Could you check a few things on this model? Use its own coordinates, in mm. Face numbers are marked on the shaded views. A direction names the side the tool comes from. Give positions to 0.01 mm unless a question says otherwise; leave off trailing zeros. Write each loop counter-clockwise with the first axis right and the second up, starting at its lowest first coordinate (ties: lowest second). Pieces come first, ordered by that corner, then holes. Notation, with made-up numbers: M 16.25,-10 L 32.25,-10 A37 cw 32.25,26 Z; hole C 0,82 d5. An arc over 180 degrees is marked long. Answer as CSV lines item,"result". Start each with the question number.
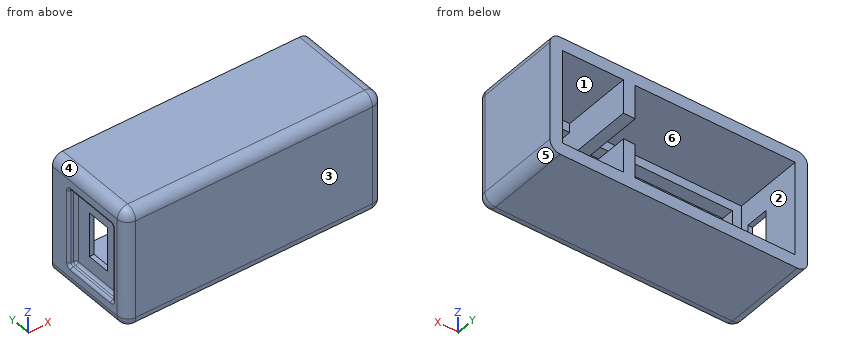
Autodesk Inventor part; units mm, degrees
ref_plane "YZ Plane" through (0, 0, 0) normal (1, 0, 0) x (0, 1, 0)
ref_plane "XZ Plane" through (0, 0, 0) normal (0, 1, 0) x (-1, 0, 0)
ref_plane "XY Plane" through (0, 0, 0) normal (0, 0, 1) x (1, 0, 0)
sketch "Sketch1" plane through (0, 0, 0) normal (0, 1, 0) x (-1, 0, 0)
  line L0 (0, 0) -> (-44.5, 0)
  line L1 (-44.5, 0) -> (-44.5, -18)
  line L2 (-44.5, -18) -> (0, -18)
  line L3 (0, -18) -> (0, 0)
  line L4 (2.4, -20.4) -> (-46.9, -20.4)
  line L5 (-46.9, -20.4) -> (-46.9, 2.4)
  line L6 (-46.9, 2.4) -> (2.4, 2.4)
  line L7 (2.4, 2.4) -> (2.4, -20.4)
  dimension "d0" = 18
  dimension "d1" = 44.5
  dimension "d2" = 2.4
extrude "Extrusion1" add sketch "Sketch1" against normal blind 2.4 contours L3 L2 L1 L0 | L4 L5 L6 L7
extrude "Extrusion2" add sketch "Sketch1" along normal blind 15.8
sketch "Sketch2" plane through (0, 0, 0) normal (0, 1, 0) x (1, 0, 0)
  line L0 (0, 0) -> (44.5, 0)
  line L1 (44.5, 0) -> (44.5, 18)
  line L2 (44.5, 18) -> (0, 18)
  line L3 (0, 18) -> (0, 0)
  line L4 (1.75, 16.25) -> (42.75, 16.25)
  line L5 (42.75, 16.25) -> (42.75, 1.75)
  line L6 (42.75, 1.75) -> (1.75, 1.75)
  line L7 (1.75, 1.75) -> (1.75, 16.25)
  line L8 (32.85, 17.25) -> (42.75, 17.25)
  line L9 (42.75, 17.25) -> (42.75, 0.75)
  line L10 (42.75, 0.75) -> (32.85, 0.75)
  line L11 (32.85, 0.75) -> (32.85, 17.25)
  line L12 (42.75, 13.5) -> (44.5, 13.5)
  line L13 (44.5, 13.5) -> (44.5, 4.5)
  line L14 (44.5, 4.5) -> (42.75, 4.5)
  line L15 (42.75, 4.5) -> (42.75, 13.5)
  line L16 (44.5, 18) -> (44.5, 0)
  point P0 (42.75, 9)
  point P1 (44.5, 9)
  point P2 (43.625, 4.5)
  point P3 (42.75, 4.5)
  point P4 (42.75, 13.5)
  dimension "d7" = 1.75
  dimension "d8" = 9.9
  dimension "d9" = 16.5
  dimension "d10" = 9
extrude "Extrusion3" add sketch "Sketch2" along normal blind 2.4 contours L3 L2 L1 L12 L5 L9 L8 L11 L4 L7 L6 L10 L14 L0 | L9 L10 L11 L6 | L4 L11 L8 L9
sketch "Sketch3" plane through (0, 2.4, 0) normal (0, 1, 0) x (1, 0, 0)
  line L0 (32.85, 0.75) -> (32.85, 17.25)
  line L1 (44.5, 4.5) -> (44.5, 0)
  line L2 (44.5, 4.5) -> (42.75, 4.5)
  line L3 (42.75, 4.5) -> (42.75, 1.75)
  line L4 (42.75, 1.75) -> (1.75, 1.75)
  line L5 (1.75, 1.75) -> (1.75, 16.25)
  line L6 (1.75, 16.25) -> (42.75, 16.25)
  line L7 (42.75, 16.25) -> (42.75, 13.5)
  line L8 (42.75, 13.5) -> (44.5, 13.5)
  line L9 (44.5, 18) -> (44.5, 13.5)
  line L10 (0, 18) -> (44.5, 18)
  line L11 (0, 0) -> (0, 18)
  line L12 (44.5, 0) -> (0, 0)
  line L13 (32.85, 18) -> (30.6, 18)
  line L14 (30.6, 18) -> (30.6, 11.5)
  line L15 (30.6, 11.5) -> (32.85, 11.5)
  line L16 (32.85, 11.5) -> (32.85, 18)
  line L17 (32.85, 0) -> (30.6, 0)
  line L18 (30.6, 0) -> (30.6, 6.5)
  line L19 (30.6, 6.5) -> (32.85, 6.5)
  line L20 (32.85, 6.5) -> (32.85, 0)
  line L21 (44.5, 0) -> (0, 0)
  line L22 (0, 18) -> (44.5, 18)
  point P0 (30.6, 1.75)
  point P1 (32.85, 1.75)
  point P2 (32.85, 16.25)
  point P3 (30.6, 16.25)
  point P4 (32.85, 0)
  dimension "d13" = 5
  dimension "d14" = 30.6
extrude "Extrusion4" add sketch "Sketch3" against normal up to surface (2.4 mm away) contours L0 L4 L18 L19 | L15 L14 L6 L0
extrude "Extrusion5" add sketch "Sketch3" along normal up to surface (13.4 mm away) contours L0 L4 L18 L19 | L15 L14 L6 L0 | L0 L20 L12 L18 L4 | L6 L14 L10 L16 L0
sketch "Sketch4" plane through (0, 2.4, 0) normal (0, 1, 0) x (1, 0, 0)
  line L0 (32.85, 18) -> (32.85, 16.25)
  line L1 (32.85, 16.25) -> (42.75, 16.25)
  line L2 (42.75, 16.25) -> (42.75, 13.5)
  line L3 (42.75, 13.5) -> (44.5, 13.5)
  line L4 (44.5, 18) -> (44.5, 13.5)
  line L5 (32.85, 18) -> (44.5, 18)
  line L6 (32.85, 1.75) -> (32.85, 0)
  line L7 (44.5, 0) -> (32.85, 0)
  line L8 (44.5, 4.5) -> (44.5, 0)
  line L9 (44.5, 4.5) -> (42.75, 4.5)
  line L10 (42.75, 4.5) -> (42.75, 1.75)
  line L11 (42.75, 1.75) -> (32.85, 1.75)
  line L12 (42.75, 16.25) -> (42.75, 18)
  line L13 (42.75, 1.75) -> (42.75, 0)
  point P0 (0, 0)
extrude "Extrusion6" add sketch "Sketch4" along normal blind 4.8 contours L5 L4 L3 L2 L12 | L10 L9 L8 L7 L13
sketch "Sketch5" plane through (-2.4, -2.4, -20.4) normal (-1, 0, 0) x (0, 0, 1)
  line L0 (20.4, 4.8) -> (2.4, 4.8)
  line L1 (7.15, 10.9) -> (15.65, 10.9)
  line L2 (15.65, 10.9) -> (15.65, 6.4)
  line L3 (15.65, 6.4) -> (7.15, 6.4)
  line L4 (7.15, 6.4) -> (7.15, 10.9)
  line L5 (11.4, 4.8) -> (11.4, 2.8169) construction
  point P0 (20.4, 2.4)
  point P1 (11.4, 6.4)
  dimension "d21" = 8.5
  dimension "d22" = 4.5
  dimension "d23" = 1.6
extrude "Extrusion7" cut sketch "Sketch5" against normal up to surface (2.4 mm away)
sketch "Sketch6" plane through (-2.4, -2.4, -20.4) normal (-1, 0, 0) x (0, 0, 1)
  line L0 (7.15, 10.9) -> (15.65, 10.9)
  line L1 (7.15, 6.4) -> (7.15, 10.9)
  line L2 (15.65, 6.4) -> (7.15, 6.4)
  line L3 (15.65, 10.9) -> (15.65, 6.4)
  line L4 (18.9, 14.15) -> (3.9, 14.15)
  line L5 (3.9, 14.15) -> (3.9, 3.15)
  line L6 (3.9, 3.15) -> (18.9, 3.15)
  line L7 (18.9, 3.15) -> (18.9, 14.15)
  point P0 (20.4, 2.4)
  dimension "d26" = 15
extrude "Extrusion8" cut sketch "Sketch6" against normal blind 1.5
fillet "Fillet1" radius 0.5 12 edges at (-1.65, 11.75, -16.5) (-1.65, 11.75, -1.5) (-1.65, 0.75, -1.5) (-1.65, 0.75, -16.5) (-2.4, 11.75, -9) (-2.4, 6.25, -16.5) (-2.4, 0.75, -9) (-2.4, 6.25, -1.5) (-0.9, 0.75, -9) (-0.9, 6.25, -16.5) (-0.9, 11.75, -9) (-0.9, 6.25, -1.5)
fillet "Fillet2" radius 2 8 edges at (22.25, -2.4, -20.4) (-2.4, -2.4, -9) (22.25, -2.4, 2.4) (46.9, -2.4, -9) (46.9, 6.7, 2.4) (46.9, 6.7, -20.4) (-2.4, 6.7, -20.4) (-2.4, 6.7, 2.4)
properties part number "rf_tester_bottom"
1. Imagine slicing it at D-D, the plane x = 39. Please give me the cut outline in (y, z), plus the area to 3 significant figures.
2. Imagine slicing it at C-C, the plane z = -15. Please give me the cut outline in (x, y), plus the area to 3 significant figures.
3. Imagine slicing it at A-A, the plane z = -7. Please give me the cut outline in (x, y).
4. Thinking about a two-plate mould opening in X: for the marked faces 1, 2, 3 and 4, which applies, pulls with the +X half, pulls with the -X half, needs draft (parallel to the pull), parting line crosses it, or undercut?
5. Imagine slicing it at B-B, the plane y = 12.75. Please give me the cut outline in (x, z).
6. Please list where these lines run through material, in increasing order: line 1 (X direction, y = 5.5, z = -14.5); line 2 (X direction, y = 13.5, z = -17); line 3 (X direction, y = 2.5, z = -9).
7. Will these pins go through, and if not, where does the flat tip stop? P1, Ø5, axis at y = 5.5, z = -10.5, coming from the -X side; P2, Ø2, axis at x = 7.5, z = -15.5, coming from the +Y side; P3, Ø0.6, axis at x = -1.5, y = 5, coming from the -Z side.
8. On a 3-axis mill with a long thin cutter (end or side, diameter ignored), from which of +Z, -Z, +X, -X, +Y, -Y can I reach the whole of each face in a straight line? I mean the marked faces 5 and 6. Say none if no direction works.
Solutions:
1,outline,"M -2.4,-18.4 A2 ccw -0.4,-20.4 L 15.8,-20.4 L 15.8,-18 L 2.4,-18 L 2.4,-16.25 L 0,-16.25 L 0,-1.75 L 2.4,-1.75 L 2.4,0 L 15.8,0 L 15.8,2.4 L -0.4,2.4 A2 ccw -2.4,0.4 Z"
1,area,"137 mm²"
2,outline,"M -2.4,-0.4 A2 ccw -0.4,-2.4 L 44.9,-2.4 A2 ccw 46.9,-0.4 L 46.9,15.8 L 44.5,15.8 L 44.5,7.2 L 42.75,7.2 L 42.75,0 L 32.85,0 L 32.85,15.8 L 30.6,15.8 L 30.6,0 L 1.75,0 L 1.75,2.4 L 0,2.4 L 0,15.8 L -2.4,15.8 L -2.4,12.25 A0.5 ccw -1.9,11.75 L -1.4,11.75 A0.5 cw -0.9,11.25 L -0.9,1.25 A0.5 cw -1.4,0.75 L -1.9,0.75 A0.5 ccw -2.4,0.25 Z"
2,area,"228 mm²"
3,outline,"M -2.4,-0.4 A2 ccw -0.4,-2.4 L 44.9,-2.4 A2 ccw 46.9,-0.4 L 46.9,15.8 L 44.5,15.8 L 44.5,0 L 1.75,0 L 1.75,2.4 L 0,2.4 L 0,4 L -0.9,4 L -0.9,1.25 A0.5 cw -1.4,0.75 L -1.9,0.75 A0.5 ccw -2.4,0.25 Z; M -2.4,12.25 A0.5 ccw -1.9,11.75 L -1.4,11.75 A0.5 cw -0.9,11.25 L -0.9,8.5 L 0,8.5 L 0,15.8 L -2.4,15.8 Z"
4,face 1,"undercut"
4,face 2,"undercut"
4,face 3,"needs draft"
4,face 4,"pulls with the -X half"
5,outline,"M -2.4,-18.4 A2 ccw -0.4,-20.4 L 44.9,-20.4 A2 ccw 46.9,-18.4 L 46.9,0.4 A2 ccw 44.9,2.4 L -0.4,2.4 A2 ccw -2.4,0.4 Z; hole M 0,-18 L 30.6,-18 L 30.6,-11.5 L 32.85,-11.5 L 32.85,-18 L 44.5,-18 L 44.5,0 L 32.85,0 L 32.85,-6.5 L 30.6,-6.5 L 30.6,0 L 0,0 Z"
6,line 1,"-0.9 to 0, 30.6 to 32.85, 42.75 to 46.9"
6,line 2,"-2.4 to 0, 30.6 to 32.85, 44.5 to 46.9"
6,line 3,"-0.9 to 0, 44.5 to 46.9"
7,P1,"x = -0.9"
7,P2,"y = 2.4"
7,P3,"z = -20.23"
8,face 5,"-Z, +X, +Y, -Y"
8,face 6,"+Y"
